Source: three-view drawing plus pictorial views. Frame: mm from the lowest corner of the part. A direction names the side the tool comes from. Give positions to 0.01 mm unless a question says otherwise; leave off trailing zeros. Loops run counter-clockwise (first coordinate to the right, second up) from the corner with the lowest first, then second, coordinate; pieces in that order, holes last. Notation, with made-up numbers: M -29.5,71 L 21.5,71 A17 cw 21.5,87 Z; hole C -30.75,46 d7. An arc over 180 degrees is marked long. Answer as a JSON object with one key per item and string values. Group by question number.
1) Section query C-C on z = 10. Return loops of the section in (x, y), plus the area to 3 significant figures.
2) Ray query, L1, parallel to Y at x = 6, z = 33.5; L2, parallel to X at y = 3.5, z = 6. Return the intervals inside material, ascending.
3) First-contact query: P1, Ø2.5, axis at x = 4, y = 4.5, coming from the -Z side. Flat tip, straight axial feed; report the tip coordinate or a pass-through.
4) Section query D-D on x = 2.5. Return loops of the section in (y, z), plus the area to 3 significant figures.
5) Access query for the marked faces 4 and 5. Directions: +Z, -Z, +X, -X, +Y, -Y. A direction counts if a zero-diameter tool reaches every point of the face in a straight line with its end or side. Return the directions, or none.
6) Section query A-A on x = 6. Return loops of the section in (y, z), plus the area to 3 significant figures.
7) Draft query along Y for the marked faces 1, 2 and 3. Return one class per face: +Y half, -Y half, draft (parallel to the pull), parting line (faces both ways), or undercut.
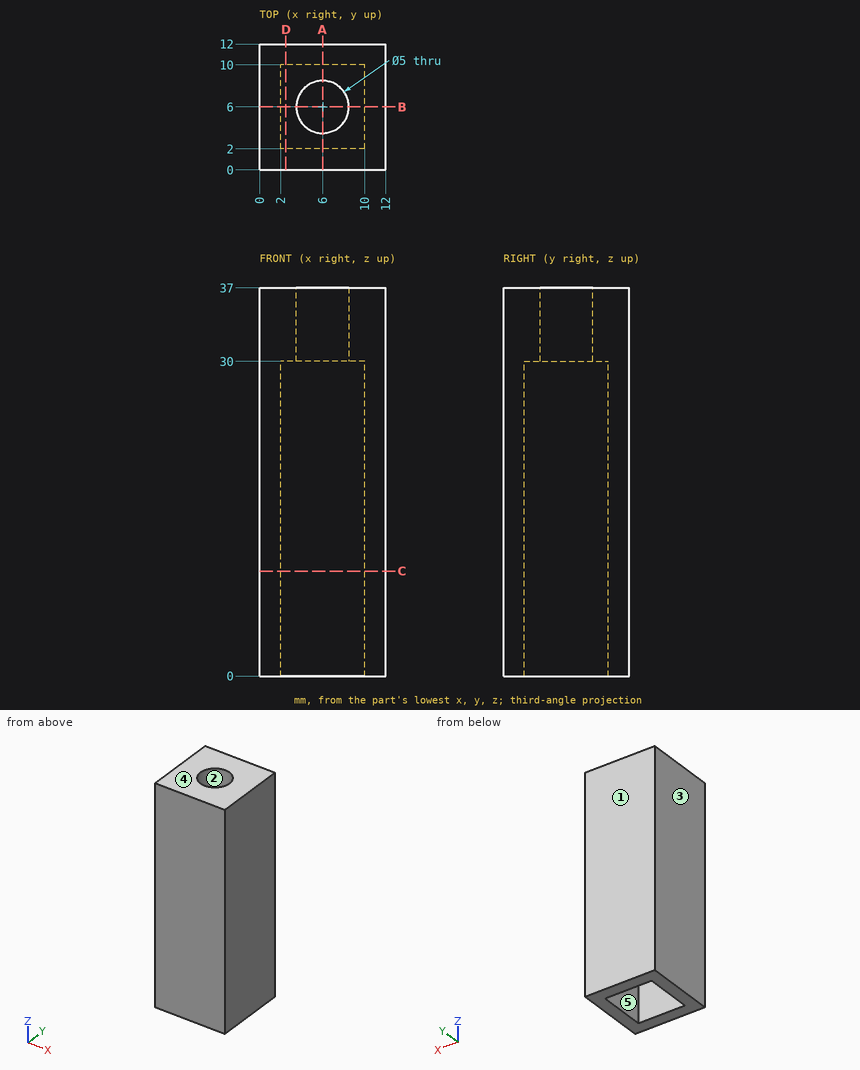
Output:
{
 "1": {"outline": "M 0,0 L 12,0 L 12,12 L 0,12 Z; hole M 2,2 L 10,2 L 10,10 L 2,10 Z", "area": "80.0 mm^2"},
 "2": {"L1": "y = 0 to 3.5, 8.5 to 12", "L2": "x = 0 to 2, 10 to 12"},
 "3": {"P1": "stops at z = 30"},
 "4": {"outline": "M 0,0 L 2,0 L 2,30 L 10,30 L 10,0 L 12,0 L 12,37 L 0,37 Z", "area": "204 mm^2"},
 "5": {"face 4": "+Z, +X, -X, +Y, -Y", "face 5": "-Z"},
 "6": {"outline": "M 0,0 L 2,0 L 2,30 L 3.5,30 L 3.5,37 L 0,37 Z; M 8.5,30 L 10,30 L 10,0 L 12,0 L 12,37 L 8.5,37 Z", "area": "169 mm^2"},
 "7": {"face 1": "+Y half", "face 2": "undercut", "face 3": "draft"}
}
